Geometry: see drawing. Coordinates: mm, zero at the bounding-box minimum. A direction names the side the tool comes from. Give positions to 0.01 mm unless a question says otherwise; leave off trailing zeros. Write each loop counter-clockwise with the first axis right and the second up, starting at its lowest first coordinate (ties: lowest second). Pieces come first, ordered by that corner, then holes. Notation, with made-up numbers: (59, -27.75) -> (78, -27.75) arc R18 ccw to (78, -10.75) -> close; hole circle Ø7 at (65, 10.25). An arc over 180 degrees is marked (long way). Answer as a JSON object with one key per item and string values. Group by question number.
Item 1: Section query B-B on y = 27.45. Return the cut outline in (x, z) (3 decimals), plus the area to 3 significant figures.
Item 2: Pull-direction query (Y, two-part tool) for the marked faces 1, 2 and 3; classes: pulls with the +Y half, pulls with the -Y half, needs draft (parallel to the pull), parting line crosses it, or undercut.
Item 3: First-contact query: pin 1 Ø6 at (x, z) = (78, 6) entering from -Y; pin 2 Ø3.5 at (x, z) = (22.5, 4) entering from +Y; pin 3 Ø6 at (y, z) = (50.5, 7.5) entering from +X. Flat tips, straight axial feed; report the tip coordinate or a pass-through.
Item 4: Section query C-C on z = 9.5. Return the cut outline in (x, y) (3 decimals).
Item 5: Section query D-D on y = 34. Return the cut outline in (x, z) (3 decimals), plus the area to 3 significant figures.
Item 6: Section query A-A on x = 85.5. Return the cut outline in (y, z).
Item 7: Ray query, probe 1 along X at (y, z) = (27.45, 3.25) (3 decimals); probe 2 along X at (y, z) = (17.5, 6.75) (3 decimals); probe 3 along Y at (x, z) = (61, 10.5). Return the intervals inside material, ascending. Write a range as from..to.
Item 8: Access query for the marked faces 4, 5 and 6. Directions: +Z, -Z, +X, -X, +Y, -Y. A direction counts if a zero-diameter tool reaches every point of the face in a straight line with its end or side. Return the directions, or none.
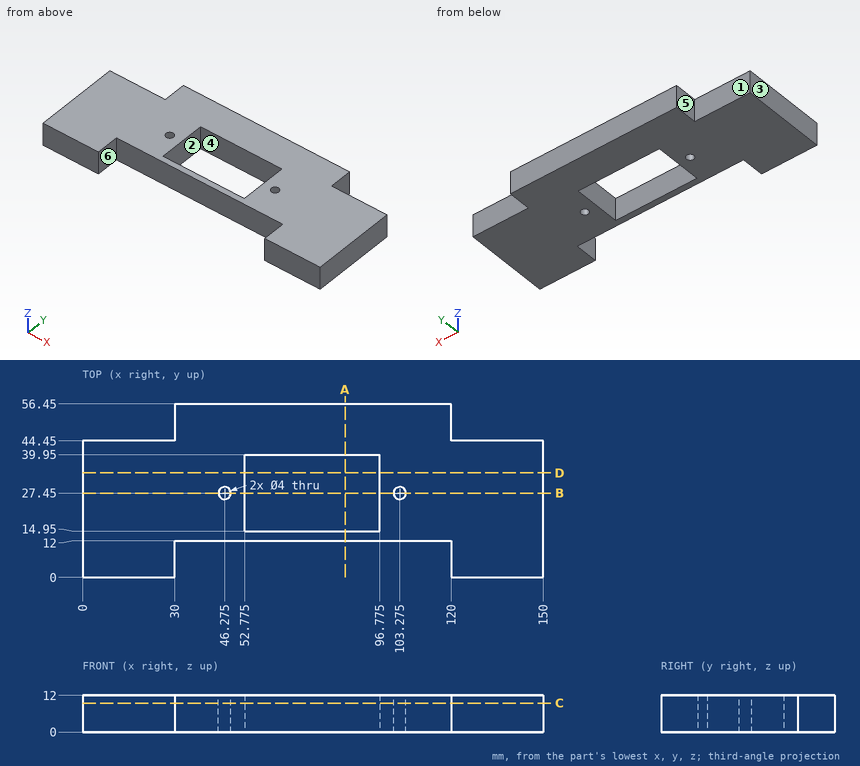
Worked answers:
{
 "1": {"outline": "(0, 0) -> (44.275, 0) -> (44.275, 12) -> (0, 12) -> close; (48.275, 0) -> (52.775, 0) -> (52.775, 12) -> (48.275, 12) -> close; (96.775, 0) -> (101.275, 0) -> (101.275, 12) -> (96.775, 12) -> close; (105.275, 0) -> (150, 0) -> (150, 12) -> (105.275, 12) -> close", "area": "1,180 mm^2"},
 "2": {"face 1": "pulls with the +Y half", "face 2": "undercut", "face 3": "needs draft"},
 "3": {"pin 1": "y = 12", "pin 2": "y = 44.45", "pin 3": "x = 120"},
 "4": {"outline": "(0, 0) -> (30, 0) -> (30, 12) -> (120, 12) -> (120, 0) -> (150, 0) -> (150, 44.45) -> (120, 44.45) -> (120, 56.45) -> (30, 56.45) -> (30, 44.45) -> (0, 44.45) -> close; hole circle Ø4 at (46.275, 27.45); hole (52.775, 14.95) -> (96.775, 14.95) -> (96.775, 39.95) -> (52.775, 39.95) -> close; hole circle Ø4 at (103.275, 27.45)"},
 "5": {"outline": "(0, 0) -> (52.775, 0) -> (52.775, 12) -> (0, 12) -> close; (96.775, 0) -> (150, 0) -> (150, 12) -> (96.775, 12) -> close", "area": "1,270 mm^2"},
 "6": {"outline": "(12, 0) -> (14.95, 0) -> (14.95, 12) -> (12, 12) -> close; (39.95, 0) -> (56.45, 0) -> (56.45, 12) -> (39.95, 12) -> close"},
 "7": {"probe 1": "0..44.275, 48.275..52.775, 96.775..101.275, 105.275..150", "probe 2": "0..52.775, 96.775..150", "probe 3": "12..14.95, 39.95..56.45"},
 "8": {"face 4": "+Z, -Z", "face 5": "+Z, -Z, -X, +Y", "face 6": "+Z, -Z, -Y"}
}
